```python
from build123d import *

# Parameters (mm, degrees)
SKETCH1_W           = 79.375
SKETCH1_H           = 23.495
BOSS_EXTRUDE1_DEPTH = 5.08
SKETCH2_W           = 79.375
SKETCH2_H           = 3.175
BOSS_EXTRUDE2_DEPTH = 25.4
SKETCH3_W           = 52.546018004
SKETCH3_H           = 5.08
BOSS_EXTRUDE3_DEPTH = 5.08
BOSS_EXTRUDE4_DEPTH = 10.16
CUT_EXTRUDE1_REACH  = 91.699
CUT_EXTRUDE2_REACH  = 91.699
FILLET2_R           = 6.35
FILLET3_R           = 6.35
FILLET4_R           = 6.35
FILLET5_R           = 6.35
BOSS_EXTRUDE6_DEPTH = 2.54
BOSS_EXTRUDE7_DEPTH = 25.4
FILLET6_R           = 6.35
FILLET7_START       = 52.546018004
FILLET7_DEPTH       = 26.828981996
FILLET7_START_2     = 5.08
FILLET7_2_DEPTH     = 6.92
FILLET8_START       = -18
FILLET8_DEPTH       = 19
FILLET9_R           = 3.175


with BuildPart() as part:
    # Sketch1 → Boss-Extrude1 (new body)
    with BuildSketch(Plane(origin=(0, 0, 0), x_dir=(1, 0, 0), z_dir=(0, 1, 0))):
        with Locations((39.6875, 11.7475)):
            Rectangle(SKETCH1_W, SKETCH1_H)
    extrude(amount=BOSS_EXTRUDE1_DEPTH)

    # Sketch2 → Boss-Extrude2 (add)
    with BuildSketch(Plane(origin=(0, 5.08, 0), x_dir=(1, 0, 0), z_dir=(0, 1, 0))):
        with Locations((39.6875, 1.5875)):
            Rectangle(SKETCH2_W, SKETCH2_H)
    extrude(amount=BOSS_EXTRUDE2_DEPTH)

    # Sketch3 → Boss-Extrude3 (add)
    with BuildSketch(Plane(origin=(0, 0, -23.495), x_dir=(-1, 0, 0), z_dir=(0, 0, -1))):
        with Locations((-26.273009002, 2.54)):
            Rectangle(SKETCH3_W, SKETCH3_H)
    extrude(amount=BOSS_EXTRUDE3_DEPTH)

    # Sketch4 → Boss-Extrude4 (add)
    with BuildSketch(Plane(origin=(0, 5.08, 0), x_dir=(1, 0, 0), z_dir=(0, 1, 0))):
        Polygon((46.196018004, 28.575), (0, 28.575), (0, 10.795), (21.397643113, 10.795), (21.397643113, 23.495), (46.196018004, 23.495), align=None)
    extrude(amount=BOSS_EXTRUDE4_DEPTH)

    # Sketch7 → Cut-Extrude1 (cut, up to next)
    with BuildSketch(Plane(origin=(0, 0, -28.575), x_dir=(-1, 0, 0), z_dir=(0, 0, -1)), mode=Mode.PRIVATE) as cut_extrude1_sk1:
        with BuildLine():
            Line((-40.146830558, 11.43), (-40.146830558, 15.24))
            Line((-40.146830558, 15.24), (-33.796830558, 15.24))
            Line((-33.796830558, 15.24), (-33.796830558, 11.43))
            ThreePointArc((-33.796830558, 11.43), (-36.971830558, 8.255), (-40.146830558, 11.43))
        make_face()
    cut_extrude1_tool1 = extrude(cut_extrude1_sk1.sketch, amount=-CUT_EXTRUDE1_REACH, mode=Mode.PRIVATE) & part.part
    add(cut_extrude1_tool1.solids().sort_by_distance((36.971831, 12.048348, -28.575))[0], mode=Mode.SUBTRACT)

    # Sketch8 → Cut-Extrude2 (cut, up to next)
    with BuildSketch(Plane.ZY, mode=Mode.PRIVATE) as cut_extrude2_sk1:
        with BuildLine():
            Line((-13.97, 11.43), (-13.97, 15.24))
            Line((-13.97, 15.24), (-20.32, 15.24))
            Line((-20.32, 15.24), (-20.32, 11.43))
            ThreePointArc((-20.32, 11.43), (-17.145, 8.255), (-13.97, 11.43))
        make_face()
    cut_extrude2_tool1 = extrude(cut_extrude2_sk1.sketch, amount=-CUT_EXTRUDE2_REACH, mode=Mode.PRIVATE) & part.part
    add(cut_extrude2_tool1.solids().sort_by_distance((0, 12.048348, -17.145))[0], mode=Mode.SUBTRACT)

    # Fillet2
    # the kernel refuses this fillet: 6.35 mm, written as the material it adds along each edge
    with BuildSketch(Plane(origin=(52.546018004, 5.08, -23.495), x_dir=(1, 0, 0), z_dir=(0, -1, 0))) as fillet2_piece_1:
        with BuildLine():
            CenterArc((6.221703947, -6.35), FILLET2_R, 90, 78.463040967)
            Line((0, -5.08), (0, 0))
            Line((0, 0), (6.221703947, 0))
        make_face()
    extrude(amount=5.08)
    # the kernel refuses this fillet: 6.35 mm, written as the material it takes off along each edge
    with BuildSketch(Plane(origin=(0, 31.115, -28.575), x_dir=(0, 0, 1), z_dir=(0, -1, 0))) as fillet2_2_piece_1:
        with BuildLine():
            CenterArc((FILLET2_R, -FILLET2_R), FILLET2_R, 90, 90)
            Line((0, -FILLET2_R), (0, 0))
            Line((0, 0), (FILLET2_R, 0))
        make_face()
    extrude(amount=46.99, mode=Mode.SUBTRACT)
    with BuildSketch(Plane(origin=(79.375, -15.875, -23.495), x_dir=(0, 0, 1), z_dir=(0, 1, 0))) as fillet2_2_piece_2:
        with BuildLine():
            CenterArc((FILLET2_R, -FILLET2_R), FILLET2_R, 90, 90)
            Line((0, -FILLET2_R), (0, 0))
            Line((0, 0), (FILLET2_R, 0))
        make_face()
    extrude(amount=36.83, mode=Mode.SUBTRACT)

    # Fillet3
    fillet3_edges = [part.edges().sort_by_distance(p)[0] for p in [
        (52.546018004, 2.54, -28.575),
    ]]
    fillet(fillet3_edges, radius=FILLET3_R)

    # Fillet4
    fillet4_edges = [part.edges().sort_by_distance(p)[0] for p in [
        (46.196018004, 5.08, -26.035),
    ]]
    fillet(fillet4_edges, radius=FILLET4_R)

    # Fillet5
    # the kernel refuses this fillet: 6.35 mm, written as the material it takes off along each edge
    with BuildSketch(Plane(origin=(46.196018004, 15.24, -8.261480267), x_dir=(-1, 0, 0), z_dir=(0, 0, -1))) as fillet5_piece_1:
        with BuildLine():
            CenterArc((6.093407893, -6.35), FILLET5_R, 90, 78.463040967)
            Line((-0.128296053, -5.08), (-0.750466448, -4.953))
            ThreePointArc((-0.750466448, -4.953), (-0.635, -3.81), (-0.635, 0))
            Line((-0.635, 0), (0, 0.635))
            Line((0, 0.635), (6.093407893, 0.635))
            Line((6.093407893, 0.635), (6.093407893, 0))
        make_face()
    extrude(amount=35.547039467, mode=Mode.SUBTRACT)

    # Sketch10 → Boss-Extrude6 (add)
    with BuildSketch(Plane.ZY):
        with BuildLine():
            Line((-3.175, 5.08), (-10.795, 5.08))
            Line((-10.795, 5.08), (-10.795, 15.24))
            Line((-10.795, 15.24), (-13.97, 15.24))
            ThreePointArc((-13.97, 15.24), (-11.72493597, 16.16993597), (-10.795, 18.415))
            Line((-10.795, 18.415), (-10.795, 27.305))
            ThreePointArc((-10.795, 27.305), (-9.86506403, 29.55006403), (-7.62, 30.48))
            Line((-7.62, 30.48), (-3.175, 30.48))
            Line((-3.175, 30.48), (-3.175, 5.08))
        make_face()
    extrude(amount=-BOSS_EXTRUDE6_DEPTH)

    # Sketch11 → Boss-Extrude7 (add)
    with BuildSketch(Plane(origin=(0, 5.08, 0), x_dir=(1, 0, 0), z_dir=(0, 1, 0))):
        Polygon((79.375, 3.175), (79.375, 17.145), (52.546018004, 17.145), (52.546018004, 10.795), (76.2, 10.795), (76.2, 3.175), align=None)
    extrude(amount=BOSS_EXTRUDE7_DEPTH)

    # Fillet6
    fillet6_edges = [part.edges().sort_by_distance(p)[0] for p in [
        (52.546018004, 30.48, -13.97),
    ]]
    fillet(fillet6_edges, radius=FILLET6_R)

    # Fillet7: read off the stored shape, not the designer's step
    # Fillet7 outline → Fillet7 (add)
    with BuildSketch(Plane.YZ.offset(FILLET7_START)):
        with BuildLine():
            ThreePointArc((5.08, -23.495), (6.939871939, -19.004871939), (11.43, -17.145))
            Line((11.43, -17.145), (5.08, -17.145))
            Line((5.08, -17.145), (5.08, -23.495))
        make_face()
    extrude(amount=FILLET7_DEPTH)

    # Fillet7 2 outline → Fillet7 2 (cut)
    with BuildSketch(Plane(origin=(0, 0, 0), x_dir=(1, 0, 0), z_dir=(0, 1, 0)).offset(FILLET7_START_2)):
        with BuildLine():
            Line((72, 23.495), (73.025, 23.495))
            ThreePointArc((73.025, 23.495), (77.515129122, 21.635126999), (79.375, 17.144996999))
            Line((79.375, 17.144996999), (79.374999459, 16))
            Line((79.374999459, 16), (81, 16))
            Line((81, 16), (81, 25))
            Line((81, 25), (72, 25))
            Line((72, 25), (72, 23.495))
        make_face()
    extrude(amount=FILLET7_2_DEPTH, mode=Mode.SUBTRACT)

    # Fillet8: read off the stored shape, not the designer's step
    # Fillet8 outline → Fillet8 (cut)
    with BuildSketch(Plane.XY.offset(FILLET8_START)):
        with BuildLine():
            Line((79.375, 30.48), (76.2, 30.48))
            ThreePointArc((76.2, 30.48), (78.44506403, 29.55006403), (79.375, 27.305))
            Line((79.375, 27.305), (79.375, 30.48))
        make_face()
    extrude(amount=FILLET8_DEPTH, mode=Mode.SUBTRACT)

    # Fillet9
    fillet9_edges = [part.edges().sort_by_distance(p)[0] for p in [
        (38.1, 30.48, 0),
        (79.375, 13.6525, 0),
        (0, 15.24, 0),
        (78.44506403, 29.55006403, 0),
    ]]
    fillet(fillet9_edges, radius=FILLET9_R - 0.0001)  # a hair under: the kernel refuses the full size


solid = part.part
```
Model file for the job. Use its own axes, mm. A direction names the side the tool comes from. Give positions to 0.01 mm unless a question says otherwise; leave off trailing zeros. Write each loop counter-clockwise with the first axis right and the second up, starting at its lowest first coordinate (ties: lowest second). Pieces come first, ordered by that corner, then holes. Notation, with made-up numbers: (-11, 3) - (-7, 3) arc R25 cw to (-7, 33) - close; hole circle Ø4 at (41.5, 47.5). An arc over 180 degrees is marked (long way). One line per question, with ' | ' between items. Start each with the question number.
(1) Wall check: line 1 along Z through (x, y) = (20, 13.5) (3 decimals); line 2 along Z through (x, y) = (20, 6) (3 decimals); line 3 along X through (y, z) = (13, -5) (3 decimals). Give the ranges that are in metal, low to high. Write a range as from..to.
(2) Pin check, flat tips, straight feed: P1, Ø2.5, axis at x = 16, z = -22.5, coming from the +Y side; P2, Ø1.3, axis at x = 1.5, y = 21.5, coming from the -Z side (3 decimals); P3, Ø1.9, axis at x = 54.5, z = -24.5, coming from the +Y side. Stop position of each tip, or through.
(3) Slice it at C-C on y = 13. Write the cut outline in (x, z) (3 decimals), plus the area to 3 significant figures.
(4) Slice it at D-D on z = -15.25. Write the cut outline in (x, y) (3 decimals).
(5) 3-axis set-ups, long thin cutter, end or side, ignore diameter. For faces 1 (the face through (66, 21, -17.145)), 2 (the face through (1, 23, -10.795)), 3 (the face through (65.773, 6.891, -19.055)): which of +Z, -Z, +X, -X, +Y, -Y reach the whole face in a straight line?
(6) Two-plate mould, pull along Z, no slides. Class faces 4 (the face through (1.252, 16.145, -11.75)), 5 (the face through (36.902, 8.256, -26.071)), 6 (the face through (64, 18, -10.795)): +Z half, -Z half, draft (parallel to the pull), parting line (faces both ways), or undercut.
(7) Slice it at B-B on z = -24.5. Write the cut outline in (x, y) (3 decimals).
Results below:
1) line 1: -28.575..-20.32, -13.97..-10.795, -3.175..0 | line 2: -28.575..-10.795, -3.175..0 | line 3: 0..2.54, 76.2..79.375
2) P1: y = 15.24 | P2: z = -10.795 | P3: y = 5.08
3) outline: (0, -22.225) arc R6.35 ccw to (6.35, -28.575) - (33.797, -28.575) - (33.797, -23.495) - (21.398, -23.495) - (21.398, -20.32) - (0, -20.32) - close; (0, -13.97) - (21.398, -13.97) - (21.398, -10.795) - (2.54, -10.795) - (2.54, -3.175) - (76.2, -3.175) - (76.2, -10.795) - (52.546, -10.795) - (52.546, -17.145) - (79.375, -17.145) - (79.375, -3.175) arc R3.175 ccw to (76.2, 0) - (3.175, 0) arc R3.175 ccw to (0, -3.175) - close; (40.147, -28.575) - (44.943, -28.575) - (44.943, -23.495) - (40.147, -23.495) - close | area: 785 mm^2
4) outline: (0, 0) - (79.375, 0) - (79.375, 27.305) arc R3.175 ccw to (76.2, 30.48) - (58.896, 30.48) arc R6.35 ccw to (52.546, 24.13) - (52.546, 5.08) - (21.398, 5.08) - (21.398, 8.883) - (0, 8.883) - close
5) face 1: -Z, +X, -X, +Y | face 2: -Z, -X, +Y | face 3: -Z, +X, +Y
6) face 4: -Z half | face 5: draft | face 6: undercut
7) outline: (0.422, 0) - (55.339, 0) - (55.339, 5.08) - (52.546, 5.08) arc R6.35 cw to (46.324, 10.16) arc R6.35 ccw to (40.147, 15.24) - (40.147, 11.43) arc R3.175 cw to (33.797, 11.43) - (33.797, 15.24) - (0.422, 15.24) - close
